```python
from build123d import *

# Parameters (mm, degrees)
F1_DEPTH = 0.635
F3_SIZE  = 0.762
F4_R     = 1.778


with BuildPart() as f1:
    # F0 (on Top) → F1 (new body)
    with BuildSketch(Plane.XY):
        with BuildLine():
            ThreePointArc((-0.127, -4.4685956586), (-4.4699488919, 0.0635064084), (0, 4.4704))
            Line((0, 4.4704), (0, 5.2705))
            ThreePointArc((0, 5.2705), (-4.6779281786, 2.4279946882), (-4.3100217321, -3.0334605518))
            ThreePointArc((-4.3100217321, -3.0334605518), (-3.0676623044, -4.285745937), (-1.4816672103, -5.057947462))
            ThreePointArc((-1.4816672103, -5.057947462), (-1.0252949469, -4.933284971), (-0.6563876884, -5.2294670333))
            ThreePointArc((-0.6563876884, -5.2294670333), (-0.3921915118, -5.2558877526), (-0.127, -5.2689696573))
            Line((-0.127, -5.2689696573), (-0.127, -4.9438178115))
            Line((-0.127, -4.9438178115), (-0.127, -4.4685956586))
        make_face()
        with BuildLine():
            ThreePointArc((-1.4816672103, -5.057947462), (-3.0676623044, -4.285745937), (-4.3100217321, -3.0334605518))
            Line((-4.3100217321, -3.0334605518), (-2.032, -6.2701346419))
            Line((-2.032, -6.2701346419), (-0.127, -6.2701346419))
            Line((-0.127, -6.2701346419), (-0.127, -5.2689696573))
            ThreePointArc((-0.127, -5.2689696573), (-0.3921915118, -5.2558877526), (-0.6563876884, -5.2294670333))
            ThreePointArc((-0.6563876884, -5.2294670333), (-0.6221376368, -5.333847732), (-0.6105490096, -5.4430910386))
            ThreePointArc((-0.6105490096, -5.4430910386), (-1.3418027236, -5.9193216797), (-1.4816672103, -5.057947462))
        make_face()
    extrude(amount=F1_DEPTH)

    # F2: F1 across plane


with BuildPart() as f1_1:
    add(f1.part)
    add(f1.part.mirror(Plane.YZ))

    # F3
    f3_edges = [f1_1.edges().sort_by_distance(p)[0] for p in [
        (-2.032, -6.270135, 0.3175),
        (2.032, -6.270135, 0.3175),
    ]]
    chamfer(f3_edges, length=F3_SIZE)

    # F4
    f4_edges = [f1_1.edges().sort_by_distance(p)[0] for p in [
        (-1.27, -6.270135, 0.3175),
        (-2.470573, -5.646999, 0.3175),
        (1.27, -6.270135, 0.3175),
        (2.470573, -5.646999, 0.3175),
    ]]
    fillet(f4_edges, radius=F4_R)


solid = f1_1.part
```
The model under review builds one solid part; all positions refer to its coordinate system, in mm. Give positions to 0.01 mm unless a question says otherwise; leave off trailing zeros. Write each loop counter-clockwise with the first axis right and the second up, starting at its lowest first coordinate (ties: lowest second). Pieces come first, ordered by that corner, then holes. Notation, with made-up numbers: (71.5, 48.5) - (98.5, 48.5) arc R10 ccw to (98.5, 61.5) - close; hole circle Ø10 at (60, -27.75). An arc over 180 degrees is marked (long way). Answer in a Markdown table with one row per item. Add a question column.
1. Insertion check: P1, Ø0.9, axis at x = -1.13, y = -5.44, coming from the -Z side. The pin has a flat end and moves straight along its axis. Give the tip position at first contact, or say it passes through.
2. Wall thickness on line 1 along Y through (x, z) = (-1.5, 0.5); line 2 along Y through (x, z) = (1, 0.2); line 3 along Y through (x, z) = (3.25, 0.2): over which ranges is each line inside the solid? List them lowest first. Write a range as [from, to].
3. We need section D-D on x = -2.5. Write out the cut boundary in (y, z) (3 decimals).
4. We need section B-B on z = 0.1. Write out the cut boundary in (x, y), then the cut area to 3 significant figures.
5. We need section C-C on x = -1. Write out the cut boundary in (y, z) (3 decimals).
6. We need section A-A on y = 0. Write out the cut boundary in (x, z) (1 decimal).
Ans:
| question | item | result |
|---|---|---|
| 1 | P1 | passes through |
| 2 | line 1 | y = [-6.14, -5.81], [-5.08, -4.21], [4.21, 5.05] |
| 2 | line 2 | y = [-6.26, -5.95], [-4.94, -4.36], [4.36, 5.17] |
| 2 | line 3 | y = [-4.54, -3.07], [3.07, 4.15] |
| 3 | outline | (-5.549, 0) - (-3.706, 0) - (-3.706, 0.635) - (-5.549, 0.635) - close; (3.706, 0) - (4.64, 0) - (4.64, 0.635) - (3.706, 0.635) - close |
| 4 | outline | (-4.31, -3.03) - (-2.72, -5.29) arc R1.78 ccw to (-2.09, -5.85) - (-1.66, -6.07) arc R1.78 ccw to (-0.84, -6.27) - (-0.13, -6.27) - (-0.13, -4.47) arc R4.47 cw (long way) to (0.13, -4.47) - (0.13, -6.27) - (0.84, -6.27) arc R1.78 ccw to (1.66, -6.07) - (2.09, -5.85) arc R1.78 ccw to (2.72, -5.29) - (4.31, -3.03) arc R5.27 ccw (long way) to start; hole circle Ø1.04 at (-1.13, -5.44); hole circle Ø1.04 at (1.13, -5.44) |
| 4 | area | 28.8 mm^2 |
| 5 | outline | (-6.263, 0) - (-5.947, 0) - (-5.947, 0.635) - (-6.263, 0.635) - close; (-4.939, 0) - (-4.357, 0) - (-4.357, 0.635) - (-4.939, 0.635) - close; (4.357, 0) - (5.175, 0) - (5.175, 0.635) - (4.357, 0.635) - close |
| 6 | outline | (-5.3, 0) - (-4.5, 0) - (-4.5, 0.6) - (-5.3, 0.6) - close; (4.5, 0) - (5.3, 0) - (5.3, 0.6) - (4.5, 0.6) - close |
